Can you work these out from the model? Positions are in its coordinate system, mm. A direction names the side the tool comes from. Round coordinates to 2 decimals unless told otherwise and drop trailing zeros. Loops run counter-clockwise (first coordinate to the right, second up) from the corner with the lowest first, then second, coordinate; pieces in that order, holes last. Notation, with made-up numbers: (-2, -30) -> (4, -30) arc R13 cw to (4, -8) -> close; hole circle Ø11 at (44, 26). An arc over 180 degrees is marked (long way). Answer as a JSON object with one key per item and string values.
```python
from build123d import *

# Parameters (mm, degrees)
EXTRUDE_1_DEPTH     = 1.45
CUT_EXTRUDE_1_REACH = 4.9
SKETCH_2_R          = 1.6
SKETCH_3_R          = 2
CUT_EXTRUDE_2_DEPTH = 10
SKETCH_4_R          = 0.6
CUT_EXTRUDE_3_DEPTH = 10


with BuildPart() as part:
    # 草图1 → 凸台-拉伸1 (new body, symmetric)
    with BuildSketch(Plane.XY):
        with BuildLine():
            Line((32.2, 68.7), (34.8, 68.7))
            ThreePointArc((34.8, 68.7), (34.941421356, 68.758578644), (35, 68.9))
            Line((35, 68.9), (35, 70.15))
            ThreePointArc((35, 70.15), (35.146446609, 70.503553391), (35.5, 70.65))
            Line((35.5, 70.65), (37.5, 70.65))
            ThreePointArc((37.5, 70.65), (37.853553391, 70.503553391), (38, 70.15))
            Line((38, 70.15), (38, 44.35))
            ThreePointArc((38, 44.35), (37.853553391, 43.996446609), (37.5, 43.85))
            Line((37.5, 43.85), (35.5, 43.85))
            ThreePointArc((35.5, 43.85), (35.146446609, 43.996446609), (35, 44.35))
            Line((35, 44.35), (35, 45.6))
            ThreePointArc((35, 45.6), (34.941421356, 45.741421356), (34.8, 45.8))
            Line((34.8, 45.8), (32.2, 45.8))
            ThreePointArc((32.2, 45.8), (32.058578644, 45.741421356), (32, 45.6))
            Line((32, 45.6), (32, -45.6))
            ThreePointArc((32, -45.6), (32.058578644, -45.741421356), (32.2, -45.8))
            Line((32.2, -45.8), (34.8, -45.8))
            ThreePointArc((34.8, -45.8), (34.941421356, -45.741421356), (35, -45.6))
            Line((35, -45.6), (35, -44.35))
            ThreePointArc((35, -44.35), (35.146446609, -43.996446609), (35.5, -43.85))
            Line((35.5, -43.85), (37.5, -43.85))
            ThreePointArc((37.5, -43.85), (37.853553391, -43.996446609), (38, -44.35))
            Line((38, -44.35), (38, -70.15))
            ThreePointArc((38, -70.15), (37.853553391, -70.503553391), (37.5, -70.65))
            Line((37.5, -70.65), (35.5, -70.65))
            ThreePointArc((35.5, -70.65), (35.146446609, -70.503553391), (35, -70.15))
            Line((35, -70.15), (35, -68.9))
            ThreePointArc((35, -68.9), (34.941421356, -68.758578644), (34.8, -68.7))
            Line((34.8, -68.7), (32.2, -68.7))
            ThreePointArc((32.2, -68.7), (32.058578644, -68.758578644), (32, -68.9))
            Line((32, -68.9), (32, -72))
            ThreePointArc((32, -72), (31.121320344, -74.121320344), (29, -75))
            Line((29, -75), (-29, -75))
            ThreePointArc((-29, -75), (-31.121320344, -74.121320344), (-32, -72))
            Line((-32, -72), (-32, -68.9))
            ThreePointArc((-32, -68.9), (-32.058578644, -68.758578644), (-32.2, -68.7))
            Line((-32.2, -68.7), (-34.8, -68.7))
            ThreePointArc((-34.8, -68.7), (-34.941421356, -68.758578644), (-35, -68.9))
            Line((-35, -68.9), (-35, -70.15))
            ThreePointArc((-35, -70.15), (-35.146446609, -70.503553391), (-35.5, -70.65))
            Line((-35.5, -70.65), (-37.5, -70.65))
            ThreePointArc((-37.5, -70.65), (-37.853553391, -70.503553391), (-38, -70.15))
            Line((-38, -70.15), (-38, -44.35))
            ThreePointArc((-38, -44.35), (-37.853553391, -43.996446609), (-37.5, -43.85))
            Line((-37.5, -43.85), (-35.5, -43.85))
            ThreePointArc((-35.5, -43.85), (-35.146446609, -43.996446609), (-35, -44.35))
            Line((-35, -44.35), (-35, -45.6))
            ThreePointArc((-35, -45.6), (-34.941421356, -45.741421356), (-34.8, -45.8))
            Line((-34.8, -45.8), (-32.2, -45.8))
            ThreePointArc((-32.2, -45.8), (-32.058578644, -45.741421356), (-32, -45.6))
            Line((-32, -45.6), (-32, 45.6))
            ThreePointArc((-32, 45.6), (-32.058578644, 45.741421356), (-32.2, 45.8))
            Line((-32.2, 45.8), (-34.8, 45.8))
            ThreePointArc((-34.8, 45.8), (-34.941421356, 45.741421356), (-35, 45.6))
            Line((-35, 45.6), (-35, 44.35))
            ThreePointArc((-35, 44.35), (-35.146446609, 43.996446609), (-35.5, 43.85))
            Line((-35.5, 43.85), (-37.5, 43.85))
            ThreePointArc((-37.5, 43.85), (-37.853553391, 43.996446609), (-38, 44.35))
            Line((-38, 44.35), (-38, 70.15))
            ThreePointArc((-38, 70.15), (-37.853553391, 70.503553391), (-37.5, 70.65))
            Line((-37.5, 70.65), (-35.5, 70.65))
            ThreePointArc((-35.5, 70.65), (-35.146446609, 70.503553391), (-35, 70.15))
            Line((-35, 70.15), (-35, 68.9))
            ThreePointArc((-35, 68.9), (-34.941421356, 68.758578644), (-34.8, 68.7))
            Line((-34.8, 68.7), (-32.2, 68.7))
            ThreePointArc((-32.2, 68.7), (-32.058578644, 68.758578644), (-32, 68.9))
            Line((-32, 68.9), (-32, 72))
            ThreePointArc((-32, 72), (-31.121320344, 74.121320344), (-29, 75))
            Line((-29, 75), (29, 75))
            ThreePointArc((29, 75), (31.121320344, 74.121320344), (32, 72))
            Line((32, 72), (32, 68.9))
            ThreePointArc((32, 68.9), (32.058578644, 68.758578644), (32.2, 68.7))
        make_face()
    extrude(amount=EXTRUDE_1_DEPTH, both=True)

    # 草图2 → 切除-拉伸1 (cut, up to next)
    with BuildSketch(Plane(origin=(0, 0, -1.45), x_dir=(-1, 0, 0), z_dir=(0, 0, -1)), mode=Mode.PRIVATE) as cut_extrude_1_sk1:
        with Locations((23.8, 8.34)):
            Circle(SKETCH_2_R)
    cut_extrude_1_tool1 = extrude(cut_extrude_1_sk1.sketch, amount=-CUT_EXTRUDE_1_REACH, mode=Mode.PRIVATE) & part.part
    add(cut_extrude_1_tool1.solids().sort_by_distance((-23.8, 8.34, -1.45))[0], mode=Mode.SUBTRACT)
    # 草图2 → 切除-拉伸1 (cut, up to next)
    with BuildSketch(Plane(origin=(0, 0, -1.45), x_dir=(-1, 0, 0), z_dir=(0, 0, -1)), mode=Mode.PRIVATE) as cut_extrude_1_sk2:
        with Locations((8.56, -42.46)):
            Circle(SKETCH_2_R)
    cut_extrude_1_tool2 = extrude(cut_extrude_1_sk2.sketch, amount=-CUT_EXTRUDE_1_REACH, mode=Mode.PRIVATE) & part.part
    add(cut_extrude_1_tool2.solids().sort_by_distance((-8.56, -42.46, -1.45))[0], mode=Mode.SUBTRACT)
    # 草图2 → 切除-拉伸1 (cut, up to next)
    with BuildSketch(Plane(origin=(0, 0, -1.45), x_dir=(-1, 0, 0), z_dir=(0, 0, -1)), mode=Mode.PRIVATE) as cut_extrude_1_sk3:
        with Locations((-19.38, -42.46)):
            Circle(SKETCH_2_R)
    cut_extrude_1_tool3 = extrude(cut_extrude_1_sk3.sketch, amount=-CUT_EXTRUDE_1_REACH, mode=Mode.PRIVATE) & part.part
    add(cut_extrude_1_tool3.solids().sort_by_distance((19.38, -42.46, -1.45))[0], mode=Mode.SUBTRACT)
    # 草图2 → 切除-拉伸1 (cut, up to next)
    with BuildSketch(Plane(origin=(0, 0, -1.45), x_dir=(-1, 0, 0), z_dir=(0, 0, -1)), mode=Mode.PRIVATE) as cut_extrude_1_sk4:
        with Locations((-24.46, 9.61)):
            Circle(SKETCH_2_R)
    cut_extrude_1_tool4 = extrude(cut_extrude_1_sk4.sketch, amount=-CUT_EXTRUDE_1_REACH, mode=Mode.PRIVATE) & part.part
    add(cut_extrude_1_tool4.solids().sort_by_distance((24.46, 9.61, -1.45))[0], mode=Mode.SUBTRACT)

    # 草图3 → 切除-拉伸2 (cut)
    with BuildSketch(Plane.XY.offset(1.45)):
        with Locations((14, 26)):
            Circle(SKETCH_3_R)
        with Locations((14, -26)):
            Circle(SKETCH_3_R)
        with Locations((-14, 26)):
            Circle(SKETCH_3_R)
        with Locations((-14, -26)):
            Circle(SKETCH_3_R)
    extrude(amount=-CUT_EXTRUDE_2_DEPTH, mode=Mode.SUBTRACT)

    # 草图4 → 切除-拉伸3 (cut)
    with BuildSketch(Plane.XY.offset(1.45)):
        with Locations((-7.23, 39)):
            Circle(SKETCH_4_R)
        with Locations((7.23, 39)):
            Circle(SKETCH_4_R)
        with BuildLine():
            Line((-9.55, 29.34), (9.55, 29.34))
            ThreePointArc((9.55, 29.34), (9.868198052, 29.208198052), (10, 28.89))
            Line((10, 28.89), (10, 28.29))
            ThreePointArc((10, 28.29), (9.868198052, 27.971801948), (9.55, 27.84))
            Line((9.55, 27.84), (-9.55, 27.84))
            ThreePointArc((-9.55, 27.84), (-9.868198052, 27.971801948), (-10, 28.29))
            Line((-10, 28.29), (-10, 28.89))
            ThreePointArc((-10, 28.89), (-9.868198052, 29.208198052), (-9.55, 29.34))
        make_face()
    extrude(amount=-CUT_EXTRUDE_3_DEPTH, mode=Mode.SUBTRACT)


solid = part.part
```
Q1. I'm going to push flat-ended pins straight in: pin 1 (1.6 mm diameter, centred on x = 36, z = 0, fed in from +Y); pin 2 (1.5 mm diameter, centred on y = 16.5, z = 0, fed in from +X); pin 3 (1.6 mm diameter, centred on x = -36.5, z = 0, fed in from -Y); pin 4 (1.4 mm diameter, centred on x = 7.23, y = 39, fed in from -Z). Where does each tip first touch, or does it pass through?
Determined:
{"pin 1": "y = 70.65", "pin 2": "x = 32", "pin 3": "y = -70.65", "pin 4": "z = -1.45"}
Q2. I want a section at D-D, the plane z = -0.8. Give the number of separate pieces and of enclosed holes in the cut face, then the cut area to 3 significant figures.
Determined:
{"separate pieces": "1", "enclosed holes": "11", "area": "10,100 mm²"}
Q3. If I drill on L1, parallel to Y at x = 7.23, z = 0.65; L2, parallel to Y at x = -14, z = 1.15; L3, parallel to X at y = 39, z = 0.5, over which ranges is the centre line in solid material (lowest first)? Write a range as [from, to].
Determined:
{"L1": "[-75, 27.84], [29.34, 38.4], [39.6, 75]", "L2": "[-75, -28], [-24, 24], [28, 75]", "L3": "[-32, -7.83], [-6.63, 6.63], [7.83, 32]"}
Q4. I want a section at A-A, the plane x = -23.8. Write out the boundary of the cut face in (y, z).
Determined:
{"outline": "(-75, -1.45) -> (6.74, -1.45) -> (6.74, 1.45) -> (-75, 1.45) -> close; (9.94, -1.45) -> (75, -1.45) -> (75, 1.45) -> (9.94, 1.45) -> close"}
Q5. I want a section at B-B, the plane x = -14. Write out the boundary of the cut face in (y, z), then the cut area to 3 significant figures.
Determined:
{"outline": "(-75, -1.45) -> (-28, -1.45) -> (-28, 1.45) -> (-75, 1.45) -> close; (-24, -1.45) -> (24, -1.45) -> (24, 1.45) -> (-24, 1.45) -> close; (28, -1.45) -> (75, -1.45) -> (75, 1.45) -> (28, 1.45) -> close", "area": "412 mm²"}
Q6. We'd pull the mould along X, two halves only. Please class faces 1 (the flat face through (1, 1, -1.45)), 2 (the flat face through (33, 68.7, 0)), 3 (the cylindrical face through (-31.1, -74.14, 0.02)): pulls with the +X half, pulls with the -X half, needs draft (parallel to the pull), parting line crosses it, or undercut.
Determined:
{"face 1": "needs draft", "face 2": "undercut", "face 3": "pulls with the -X half"}
Q7. I want a section at C-C, the plane y = 26. Write out the boundary of the cut face in (x, z), then the cut area to 3 significant figures.
Determined:
{"outline": "(-32, -1.45) -> (-16, -1.45) -> (-16, 1.45) -> (-32, 1.45) -> close; (-12, -1.45) -> (12, -1.45) -> (12, 1.45) -> (-12, 1.45) -> close; (16, -1.45) -> (32, -1.45) -> (32, 1.45) -> (16, 1.45) -> close", "area": "162 mm²"}
Q8. On a 3-axis mill with a long thin cutter (end or side, diameter ignored), from which of +Z, -Z, +X, -X, +Y, -Y can I reach the whole of each face in a straight line? I mean faces 4 (the flat face through (32, -70, 0)), 5 (the flat face through (0, 75, 0)), 6 (the flat face through (-38, -57, 0)), 7 (the flat face through (33, -45.8, 0)), 8 (the flat face through (32, 70, 0)). Say none if no direction works.
Determined:
{"face 4": "+Z, -Z, -Y", "face 5": "+Z, -Z, +X, -X, +Y", "face 6": "+Z, -Z, -X, +Y, -Y", "face 7": "+Z, -Z", "face 8": "+Z, -Z, +Y"}
